Could you check a few things on this model? Use its own coordinates, in mm. Round coordinates to 2 decimals unless told otherwise and drop trailing zeros. Loops run counter-clockwise (first coordinate to the right, second up) from the corner with the lowest first, then second, coordinate; pieces in that order, holes last. Notation, with made-up numbers: (-19.5, -36) -> (17.5, -36) arc R10 ccw to (17.5, -29) -> close; hole circle Ø2 at (-34, 78). An arc over 180 degrees is marked (long way). Put each result on its own line as item: value. Start each with the question number.
1. Imagine slicing it at B-B, the plane x = -8.75. Please give me the cut outline in (y, z) (3 decimals).
2. Imagine slicing it at C-C, the plane z = -9.5. Please give me the cut outline in (x, y) (3 decimals), and give its area (3 significant figures).
3. I'm going to push flat-ended pins straight in: P1, Ø4.5, axis at x = -10, y = 20.68, coming from the -Z side; P2, Ø6, axis at x = -10, y = -20.68, coming from the +Z side; P3, Ø4, axis at x = -9, y = -6, coming from the +Z side. Where does each tip first touch, or does it pass through?
4. I need wall thicknesses on line 1 (Y direction, x = -10, z = -10) (3 decimals); line 2 (Z direction, x = -15.75, y = -0.5); line 3 (Y direction, x = -10, z = -5.75) (1 decimal). Which ranges of each line are inside material? Lowest first, please. Write a range as [from, to].
5. Imagine slicing it at A-A, the plane z = -2.25. Please give me the cut outline in (x, y) (3 decimals), and give its area (3 significant figures).
6. Imagine slicing it at D-D, the plane x = -16.25. Please give me the cut outline in (y, z) (3 decimals).
```python
from build123d import *

# Parameters (mm, degrees)
F1_DEPTH = 20
F4_DEPTH = 25


with BuildPart() as f1:
    # F0 (on Right) → F1 (new body)
    with BuildSketch(Plane.YZ):
        with BuildLine():
            ThreePointArc((0, -11), (-7.7781745931, -7.7781745931), (-11, 0))
            Line((-11, 0), (-29.125, 0))
            Line((-29.125, 0), (-29.125, -16))
            Line((-29.125, -16), (0, -16))
            Line((0, -16), (0, -11))
        make_face()
    extrude(amount=-F1_DEPTH)

    # F3 (on offset) → F4 (cut)
    with BuildSketch(Plane.XY):
        with BuildLine():
            ThreePointArc((-10, -23.1794859892), (-8.232233047, -22.4472529422), (-7.5, -20.6794859892))
            ThreePointArc((-7.5, -20.6794859892), (-11.767766953, -18.9117190362), (-10, -23.1794859892))
        make_face()
    extrude(amount=-F4_DEPTH, mode=Mode.SUBTRACT)

    # F5: F1 across face


with BuildPart() as f1_1:
    add(f1.part)
    add(f1.part.mirror(Plane(origin=(-10, 0, -13.5), x_dir=(-1, 0, 0), z_dir=(0, 1, 0))))


solid = f1_1.part
```
Entries:
1. outline: (-29.125, -16) -> (-22.845, -16) -> (-22.845, 0) -> (-29.125, 0) -> close; (-18.514, -16) -> (18.514, -16) -> (18.514, 0) -> (11, 0) arc R11 cw to (-11, 0) -> (-18.514, 0) -> close; (22.845, -16) -> (29.125, -16) -> (29.125, 0) -> (22.845, 0) -> close
2. outline: (-20, -29.125) -> (0, -29.125) -> (0, -5.545) -> (-20, -5.545) -> close; (-20, 5.545) -> (0, 5.545) -> (0, 29.125) -> (-20, 29.125) -> close; hole circle Ø5 at (-10, -20.679); hole circle Ø5 at (-10, 20.679)
2. area: 904 mm^2
3. P1: through
3. P2: z = 0
3. P3: z = -7.55
4. line 1: [-29.125, -23.179], [-18.179, -4.583], [4.583, 18.179], [23.179, 29.125]
4. line 2: [-16, -10.99]
4. line 3: [-29.1, -23.2], [-18.2, -9.4], [9.4, 18.2], [23.2, 29.1]
5. outline: (-20, -29.125) -> (0, -29.125) -> (0, -10.767) -> (-20, -10.767) -> close; (-20, 10.767) -> (0, 10.767) -> (0, 29.125) -> (-20, 29.125) -> close; hole circle Ø5 at (-10, -20.679); hole circle Ø5 at (-10, 20.679)
5. area: 695 mm^2
6. outline: (-29.125, -16) -> (29.125, -16) -> (29.125, 0) -> (11, 0) arc R11 cw to (-11, 0) -> (-29.125, 0) -> close
